```python
from build123d import *

# Parameters (mm, degrees)
F0_W     = 28
F0_H     = 10
F0_W_2   = 10
F0_H_2   = 6
F0_H_3   = 31
F1_DEPTH = 9
F2_DEPTH = 1
F3_DEPTH = 2
F4_R     = 0.99999


# Not quite as in the source:
# - a fillet or chamfer is up to 0.001 mm smaller than in the source, because OpenCascade refuses the exact size


with BuildPart() as f1:
    # F0 (on Top) → F1 (new body)
    with BuildSketch(Plane.XY):
        with Locations((14, 36)):
            Rectangle(F0_W, F0_H)
        with Locations((7, 36)):
            Rectangle(F0_W_2, F0_H_2, mode=Mode.SUBTRACT)
        with Locations((21, 36)):
            Rectangle(F0_W_2, F0_H_2, mode=Mode.SUBTRACT)
        with Locations((7, 36)):
            Rectangle(F0_W_2, F0_H_2)
        with Locations((21, 36)):
            Rectangle(F0_W_2, F0_H_2)
        with Locations((14, 15.5)):
            Rectangle(F0_W, F0_H_3)
    extrude(amount=-F1_DEPTH)

    # F0 (on Top) → F2 (join)
    with BuildSketch(Plane.XY):
        with Locations((14, 15.5)):
            Rectangle(F0_W, F0_H_3)
    extrude(amount=F2_DEPTH)

    # F0 (on Top) → F3 (join)
    with BuildSketch(Plane.XY):
        with Locations((7, 36)):
            Rectangle(F0_W_2, F0_H_2)
        with Locations((21, 36)):
            Rectangle(F0_W_2, F0_H_2)
    extrude(amount=F3_DEPTH)

    # F4 (radius 1 in the source; OpenCascade refuses exactly that, so slightly less here)
    f4_edges = [f1.edges().sort_by_distance(p)[0] for p in [
        (12, 36, 2),
        (7, 39, 2),
        (2, 36, 2),
        (7, 33, 2),
        (21, 39, 2),
        (16, 36, 2),
        (21, 33, 2),
        (26, 36, 2),
        (0, 15.5, 1),
        (14, 0, 1),
        (28, 15.5, 1),
        (14, 31, 1),
    ]]
    fillet(f4_edges, radius=F4_R)


solid = f1.part
```
Source: CAD feature listing. Evaluate the final solid. Frame: model axes, mm. A direction names the side the tool comes from. Give positions to 0.01 mm unless a question says otherwise; leave off trailing zeros. Loops run counter-clockwise (first coordinate to the right, second up) from the corner with the lowest first, then second, coordinate; pieces in that order, holes last. Notation, with made-up numbers: M 50,-38.5 L 107,-38.5 A17 cw 107,-5.5 Z; hole C 19,-2 d4. An arc over 180 degrees is marked long. Put each result on its own line as item: value.
Q1. Pin query (flat end, axial travel): P1, Ø5, axis at x = 10, y = 15.5, coming from the +Z side; P2, Ø0.5, axis at x = 8.5, z = 0.5, coming from the -Y side; P3, Ø0.5, axis at y = 36, z = 0.5, coming from the -X side. Return the tip coordinate at first contact, or that it passes through.
Response values:
P1: stops at z = 1
P2: stops at y = 0.03
P3: stops at x = 2
Q2. Mould query, pull axis Y, two halves, no side actions, for faces 4 (the flat face through (20.9, 33, 0.5)), 5 (the cylindrical face through (7.07, 38.715, 1.699)), 6 (the flat face through (6.9, 33, 0.5)), 7 (the flat face through (14, 21, -9)). Classes: released by +Y, released by -Y, zero draft, split by the parting line, or undercut.
Response values:
face 4: undercut
face 5: released by +Y
face 6: undercut
face 7: zero draft
Q3. Line query: probe 1 along Z at (x, y) = (21, 21); probe 2 along Y at (x, z) = (11.5, 0.5); probe 3 along Z at (x, y) = (12.5, 33). Output: solid intervals per line, ascending. Write a range as [from, to].
Response values:
probe 1: z = [-9, 1]
probe 2: y = [0.13, 30.87], [33, 39]
probe 3: z = [-9, 0]
Q4. Section D-D (y = 12). Return the cut outline in (x, z), and give its area (3 significant figures).
Response values:
outline: M 0,-9 L 28,-9 L 28,0 A1 ccw 27,1 L 1,1 A1 ccw 0,0 Z
area: 280 mm²
Q5. Section B-B (y = 36). Return the cut outline in (x, z).
Response values:
outline: M 0,-9 L 28,-9 L 28,0 L 26,0 L 26,1 A1 ccw 25,2 L 17,2 A1 ccw 16,1 L 16,0 L 12,0 L 12,1 A1 ccw 11,2 L 3,2 A1 ccw 2,1 L 2,0 L 0,0 Z
Q6. Reachability of faces 1 (the cylindrical face through (14.196, 30.699, 0.715)), 2 (the flat face through (26, 36, 0.5)), 3 (the flat face through (14, 16, 1)) from +Z, -Z, +X, -X, +Y, -Y: full face, straight path, thin tool, end or side. Return the list, or none.
Response values:
face 1: +Z, +X, -X
face 2: +Z, +X, +Y
face 3: +Z, +X, -X, -Y
